```python
from build123d import *

# Parameters (mm, degrees)
BOSS_EXTRUDE1_DEPTH      = 12.5
M3_CLEARANCE_HOLE1_D     = 3.4
M3_CLEARANCE_HOLE1_DEPTH = 8.5
M3_CLEARANCE_HOLE1_TIP   = 1.021463052
M3_CLEARANCE_HOLE2_D     = 3.4
M3_CLEARANCE_HOLE2_DEPTH = 8.5
M3_CLEARANCE_HOLE2_TIP   = 1.021463052


with BuildPart() as part:
    # Sketch2 → Boss-Extrude1 (new body, symmetric)
    with BuildSketch(Plane(origin=(0, 0, 0), x_dir=(0, 0, -1), z_dir=(1, 0, 0))):
        Polygon((0, 0), (0, 4), (-35, 4), (-51.781992624, 24), (-121.647223256, 24), (-121.647223256, 20), (-53.647223256, 20), (-36.865230633, 0), align=None)
    extrude(amount=BOSS_EXTRUDE1_DEPTH, both=True)

    # M3 Clearance Hole1
    with Locations(Plane(origin=(0, 24, 0), x_dir=(1, 0, 0), z_dir=(0, 1, 0))):
        with Locations((-8.4, -90.897223256), (-8.4, -114.897223256), (8.4, -114.897223256), (8.4, -90.897223256)):
            Hole(M3_CLEARANCE_HOLE1_D / 2, depth=M3_CLEARANCE_HOLE1_DEPTH)
            with Locations((0, 0, -(M3_CLEARANCE_HOLE1_DEPTH + M3_CLEARANCE_HOLE1_TIP / 2))):  # 118° drill point
                Cone(0, M3_CLEARANCE_HOLE1_D / 2, M3_CLEARANCE_HOLE1_TIP, mode=Mode.SUBTRACT)

    # M3 Clearance Hole2
    with Locations(Plane(origin=(0, 4, 0), x_dir=(1, 0, 0), z_dir=(0, 1, 0))):
        with Locations((-10, -27.5), (10, -27.5), (10, -7.5), (-10, -7.5)):
            Hole(M3_CLEARANCE_HOLE2_D / 2, depth=M3_CLEARANCE_HOLE2_DEPTH)
            with Locations((0, 0, -(M3_CLEARANCE_HOLE2_DEPTH + M3_CLEARANCE_HOLE2_TIP / 2))):  # 118° drill point
                Cone(0, M3_CLEARANCE_HOLE2_D / 2, M3_CLEARANCE_HOLE2_TIP, mode=Mode.SUBTRACT)


solid = part.part
```
Here's how the part is built. I have some questions about the finished solid (model axes, mm). A direction names the side the tool comes from. Coordinates: 2 decimals unless noted, no trailing zeros. Order: outer loops, then holes, each group sorted by start corner. A loop starts at its lowest first (then second) coordinate and runs counter-clockwise, first axis right, second up.
Item 1: If we section it at B-B, the plane x = 5: List the corners of the cut face in (y, z) for me, then the cut area to 3 significant figures.
Response values:
outline: (0, 0) - (4, 0) - (4, 35) - (24, 51.78) - (24, 121.65) - (20, 121.65) - (20, 53.65) - (0, 36.87) - close
area: 524 mm2
Item 2: If we section it at C-C, the plane z = 60: List the corners of the cut face in (x, y) for me, then the cut area to 3 significant figures.
Response values:
outline: (-12.5, 20) - (12.5, 20) - (12.5, 24) - (-12.5, 24) - close
area: 100 mm2
Item 3: If we section it at A-A, the plane z = 27.5: List the corners of the cut face in (x, y) for me, then the cut area to 3 significant figures.
Response values:
outline: (-12.5, 0) - (-11.7, 0) - (-11.7, 4) - (-12.5, 4) - close; (-8.3, 0) - (8.3, 0) - (8.3, 4) - (-8.3, 4) - close; (11.7, 0) - (12.5, 0) - (12.5, 4) - (11.7, 4) - close
area: 72.8 mm2
Item 4: Thinking about a two-plate mould opening in X: for faces 4 (the face through (12.5, 21, 61)), 5 (the face through (-8.031, 21.972, 116.557)), 6 (the face through (0.175, 10.14, 45.374)), 7 (the face through (-12.5, 21, 61)), which applies, pulls with the +X half, pulls with the -X half, needs draft (parallel to the pull), parting line crosses it, or undercut?
Response values:
face 4: pulls with the +X half
face 5: undercut
face 6: needs draft
face 7: pulls with the -X half
Item 5: Which directions (+Z, -Z, +X, -X, +Y, -Y) give clear straight access to the entire face, cutting with the end or side of a thin tool? Please do faces 1 (the face through (0, 4, 17)), 2 (the face through (-9.63, 1.97, 9.16)), 3 (the face through (0, 20, 88)).
Response values:
face 1: -Z, +X, -X, +Y
face 2: +Y, -Y
face 3: +Z, +X, -X, -Y
Item 6: If we section it at D-D, the plane y = 18.25: List the corners of the cut face in (x, z) for me, then the cut area to 3 significant figures.
Response values:
outline: (-12.5, 46.96) - (12.5, 46.96) - (12.5, 52.18) - (-12.5, 52.18) - close
area: 131 mm2
Item 7: I'm going to push flat-ended pins straight in: pin 1 Ø3 at (x, y) = (8, 15) entering from +Z; pin 2 Ø3 at (x, y) = (8, 19.5) entering from -Z; pin 3 Ø5 at (y, z) = (17, 78) entering from -X; pin 4 Ø1 at (x, z) = (9.5, 46) entering from -Y. Where does each tip first touch, or does it pass through?
Response values:
pin 1: stops at z = 50.71
pin 2: stops at z = 46.75
pin 3: passes through
pin 4: stops at y = 10.29
Item 8: I need wall thicknesses on probe 1 along X at (y, z) = (1.8, 27.5); probe 2 along Z at (x, y) = (8.4, 22.9); probe 3 along Y at (x, z) = (2, 110). Which ranges of each line are inside material? Lowest first, please.
Response values:
probe 1: x = -12.5 to -11.7, -8.3 to 8.3, 11.7 to 12.5
probe 2: z = 50.86 to 89.2, 92.6 to 113.2, 116.6 to 121.65
probe 3: y = 20 to 24
